The listing builds one solid part. Answer for the finished solid, in the listing's coordinates (mm). A direction names the side the tool comes from. Round coordinates to 2 decimals unless told otherwise and drop trailing zeros. Write each loop counter-clockwise with the first axis right and the second up, starting at its lowest first coordinate (ties: lowest second). Pieces come first, ordered by that corner, then holes.
Item 1: Find section C-C on x = -9.5. Give the vertices of the cut face in (y, z).
Item 2: Find the intervals of material crossed by probe 1 along X at (y, z) = (-1.15, 0); probe 2 along Z at (x, y) = (-31.5, -1.8); probe 3 along X at (y, z) = (-0.95, 18), in increasing order.
Item 3: Find section D-D on x = 41. Give the vertices of the cut face in (y, z).
Item 4: Find section A-A on z = 0. Give the vertices of the cut face in (x, y).
Item 5: A tool of negligible diameter and unlimited length cuts with its end or side. For faces 4 (the face through (-16.02, -1.52, 28.28)), 5 (the face through (16.202, -1.479, -128.334)), from which of +Z, -Z, +X, -X, +Y, -Y can it reach the whole face along a straight path? Write none if from no direction.
Item 6: Each of these flat-tipped pins is pushed along its axis until it touches: pin 1 (1.5 mm diameter, centred on y = -1, z = -113, fed in from -X); pin 2 (5 mm diameter, centred on x = 27, z = 21, fed in from +Y). Where does it stop, or does it pass through?
Item 7: For a pull along X with two mould halves and no side action, classify faces 1 (the face through (-1, -3, -50)), 2 (the face through (-16.308, -1.479, -126.281)), 3 (the face through (16.02, -1.52, -28.28)) as +X half, -X half, draft (parallel to the pull), parting line (faces both ways), or undercut.
Item 8: Find section B-B on y = -1.45. Give the vertices of the cut face in (x, z).
```python
from build123d import *

# Parameters (mm, degrees)
F1_DEPTH = 3
F3_DEPTH = 25


with BuildPart() as f1:
    # F0 (on Front) → F1 (new body)
    with BuildSketch(Plane.XZ):
        with BuildLine():
            ThreePointArc((20.026396, -53.972799), (24.540831, -42.310868), (35.099057, -35.609777))
            ThreePointArc((35.099057, -35.609777), (0, 50), (-35.099057, -35.609777))
            ThreePointArc((-35.099057, -35.609777), (-24.540831, -42.310868), (-20.026396, -53.972799))
            Line((-20.026396, -53.972799), (-12.483503, -200.642001))
            ThreePointArc((-12.483503, -200.642001), (0, -212.5), (12.483503, -200.642001))
            Line((12.483503, -200.642001), (20.026396, -53.972799))
        make_face()
    extrude(amount=F1_DEPTH)

    # F2 (on face) → F3 (cut)
    with BuildSketch(Plane.XZ.offset(3)):
        Polygon((-32.5, 18.763884), (-32.5, -18.763884), (0, -37.527767), (32.5, -18.763884), (32.5, 18.763884), (0, 37.527767), align=None)
    extrude(amount=-F3_DEPTH, mode=Mode.SUBTRACT)


solid = f1.part
```
Check values:
1. outline: (-3, -208.12) - (0, -208.12) - (0, -32.04) - (-3, -32.04) - close; (-3, 32.04) - (0, 32.04) - (0, 49.09) - (-3, 49.09) - close
2. probe 1: x = -50 to -32.5, 32.5 to 50
2. probe 2: z = -36.9 to -19.34, 19.34 to 38.83
2. probe 3: x = -46.65 to -32.5, 32.5 to 46.65
3. outline: (-3, -28.62) - (0, -28.62) - (0, 28.62) - (-3, 28.62) - close
4. outline: (-50, -3) - (-32.5, -3) - (-32.5, 0) - (-50, 0) - close; (32.5, -3) - (50, -3) - (50, 0) - (32.5, 0) - close
5. face 4: +Y, -Y
5. face 5: -Z, +X, +Y, -Y
6. pin 1: stops at x = -17.03
6. pin 2: stops at y = 0
7. face 1: draft
7. face 2: -X half
7. face 3: undercut
8. outline: (-35.1, -35.61) arc R20 cw to (-20.03, -53.97) - (-12.48, -200.64) arc R12.5 ccw to (12.48, -200.64) - (20.03, -53.97) arc R20 cw to (35.1, -35.61) arc R50 ccw (long way) to start; hole (-32.5, -18.76) - (0, -37.53) - (32.5, -18.76) - (32.5, 18.76) - (0, 37.53) - (-32.5, 18.76) - close
